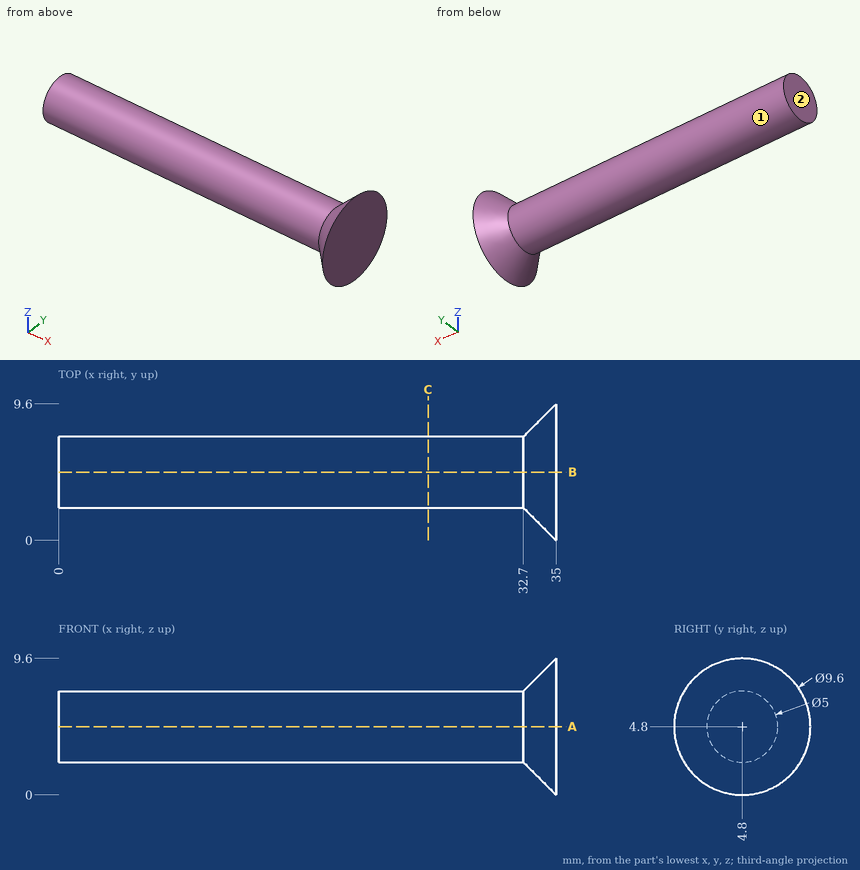
Could you check a few things on this drawing? It's one solid part, dimensions in mm from its lowest x, y, z. A direction names the side the tool comes from. Round coordinates to 2 decimals unless told otherwise and drop trailing zeros. Order: outer loops, then holes, each group sorted by start corner. A loop starts at its lowest first (then second) coordinate and runs counter-clockwise, first axis right, second up.
(1) Please list where these lines run through material, in increasing order: line 1 along Z through (x, y) = (21, 5); line 2 along Y through (x, z) = (28.5, 2.5); line 3 along X through (y, z) = (5.5, 2.25).
Response values:
line 1: z = 2.31 to 7.29
line 2: y = 3.82 to 5.78
line 3: x = 32.84 to 35
(2) I'm going to push flat-ended pins straight in: pin 1 (5 mm diameter, centred on x = 9, y = 1.5, fed in from +Z); pin 2 (1 mm diameter, centred on x = 24, y = 4.5, fed in from -Z); pin 3 (4 mm diameter, centred on x = 21, y = 5, fed in from +Z). Where does each tip first touch, or does it pass through?
Response values:
pin 1: stops at z = 7.17
pin 2: stops at z = 2.3
pin 3: stops at z = 7.3
(3) Imagine slicing it at A-A (z = 4.8). Write out the boundary of the cut face in (x, y).
Response values:
outline: (0, 2.3) - (32.7, 2.3) - (35, 0) - (35, 9.6) - (32.7, 7.3) - (0, 7.3) - close
(4) Which directions (+Z, -Z, +X, -X, +Y, -Y) give clear straight access to the entire face, cutting with the end or side of a thin tool? Please do the marked faces 1 and 2.
Response values:
face 1: -X
face 2: +Z, -Z, -X, +Y, -Y
(5) Imagine slicing it at C-C (x = 26). Write out the boundary of the cut face in (y, z).
Response values:
outline: circle Ø5 at (4.8, 4.8)
